Check sheet for the modelled part. Datum: model origin and axes. Units: mm. Coordinates: 2 decimals unless noted, no trailing zeros. Order: outer loops, then holes, each group sorted by start corner. A loop starts at its lowest first (then second) coordinate and runs counter-clockwise, first axis right, second up.
1. Cross-section at B-B (y = 1.8). Enter the section's corners in (x, z).
2. Draft check along X on faces 1 (the flat face through (1.3, -1.3, 0)), 2 (the cylindrical face through (-0.07, -1.5, 3.04)), 3 (the cylindrical face through (-0.07, 1.5, 26.96)), 4 (the cylindrical face through (-3, 0, 15)). Enter one of: released by +X, released by -X, zero draft, split by the parting line, or undercut.
3. Cross-section at D-D (x = -1.9). Enter the section's corners in (y, z).
4. Thickness scan on line 1 (Y direction, x = 0, z = 25.9); line 2 (X direction, y = -2.6, z = 19.5); line 3 (X direction, y = 0.2, z = 1.75). Record the ranges inside material, lowest first.
5. Gauge pin test, flat end, axial feed: pin 1 Ø1.8 at (x, y) = (0, 0) entering from +Z. Record the tip position at first contact, or that the pin passes through.
6. Cross-section at C-C (z = 22.25). Enter the section's corners in (x, y), then the cut area to 3 significant figures.
7. Cross-section at A-A (z = 5). Enter the section's corners in (x, y), then the cut area to 3 significant figures.
Autodesk Inventor part; units mm, degrees
ref_plane "YZ Plane" through (0, 0, 0) normal (1, 0, 0) x (0, 1, 0)
ref_plane "XZ Plane" through (0, 0, 0) normal (0, 1, 0) x (-1, 0, 0)
ref_plane "XY Plane" through (0, 0, 0) normal (0, 0, 1) x (1, 0, 0)
sketch "スケッチ1" plane through (0, 0, 0) normal (0, 0, 1) x (1, 0, 0)
  circle A0 centre (0, 0) radius 3
  dimension "d0" = 6
extrude "押し出し1" add sketch "スケッチ1" along normal blind 30
hole "穴1" at (0, 0, 0) direction (0, 0, 1) diameter 3 depth 6 tip angle 118
sketch "スケッチ2" plane through (0, 0, 30) normal (0, 0, 1) x (1, 0, 0)
  circle A0 centre (0, 0) radius 3
hole "穴2" at (0, 0, 30) direction (0, 0, -1) diameter 3 depth 6 tip angle 118
properties part number "スペーサ　m3-l30" material "アルミニウム 2014-T4"
Data:
1. outline: (-2.4, 0) - (2.4, 0) - (2.4, 30) - (-2.4, 30) - close
2. face 1: zero draft
2. face 2: undercut
2. face 3: undercut
2. face 4: split by the parting line
3. outline: (-2.32, 0) - (2.32, 0) - (2.32, 30) - (-2.32, 30) - close
4. line 1: y = -3 to -1.5, 1.5 to 3
4. line 2: x = -1.5 to 1.5
4. line 3: x = -2.99 to -1.49, 1.49 to 2.99
5. pin 1: stops at z = 23.64
6. outline: circle Ø6 at (0, 0)
6. area: 28.3 mm2
7. outline: circle Ø6 at (0, 0); hole circle Ø3 at (0, 0)
7. area: 21.2 mm2
